Could you check a few things on this model? Use its own coordinates, in mm. A direction names the side the tool comes from. Round coordinates to 2 decimals unless told otherwise and drop trailing zeros. Loops run counter-clockwise (first coordinate to the right, second up) from the corner with the lowest first, then second, coordinate; pieces in that order, holes last. Notation, with made-up numbers: (4.5, 85.5) -> (51.5, 85.5) arc R21 ccw to (51.5, 113.5) -> close; hole circle Ø10 at (34, -19). An arc over 180 degrees is marked (long way). Write each question's results on one line, items separated by ' | '.
from build123d import *

# Parameters (mm, degrees)
F1_DEPTH = 7.62
F2_DEPTH = 25.4
F4_DEPTH = 25.4
F6_DEPTH = 25.4


with BuildPart() as f1:
    # F0 (on Front) → F1 (new body)
    with BuildSketch(Plane.XZ):
        Polygon((0, -4.6985740773), (0, 0), (-4.4972063042, 0), (-18.1230716407, 0), align=None)
        Polygon((4.698574543, 0), (0, 0), (0, -4.6985740773), (4.698574543, -4.6985740773), (18.9285408705, 0), (10.8738420531, 0), align=None)
        Polygon((-4.4972063042, 0), (0, 0), (4.698574543, 0), (4.698574543, 44.1665910184), (0, 56.5171316266), (-4.4972063042, 43.0926345289), (-4.4972063042, 26.4462586492), align=None)
        with BuildLine():
            Line((4.698574543, -4.6985740773), (0, -4.6985740773))
            Line((0, -4.6985740773), (-4.4972063042, -4.6985740773))
            Line((-4.4972063042, -4.6985740773), (-4.4972063042, -7.9204533249))
            add(Edge.make_bspline(
                [(-4.4972063042, -7.9204533249), (-3.0188959312, -8.9298356018), (-0.076765682, -10.9387061232), (3.1120295895, -9.4610912419), (4.698574543, -8.7259225547)],
                knots=[0, 0, 0, 0, 0.5024625859, 1, 1, 1, 1], degree=3))
            Line((4.698574543, -8.7259225547), (4.698574543, -4.6985740773))
        make_face()
        Polygon((-4.4972063042, -4.6985740773), (0, -4.6985740773), (-18.1230716407, 0), (-8.9944126084, -4.6985740773), align=None)
        Polygon((18.9285408705, 0), (4.698574543, -4.6985740773), (10.8738420531, -4.6985740773), align=None)
        with BuildLine():
            add(Edge.make_bspline(
                [(-4.4972063042, -7.9204533249), (-3.0188959312, -8.9298356018), (-0.076765682, -10.9387061232), (3.1120295895, -9.4610912419), (4.698574543, -8.7259225547)],
                knots=[0, 0, 0, 0, 0.5024625859, 1, 1, 1, 1], degree=3))
            Line((-4.4972063042, -7.9204533249), (-4.4972063042, -12.2162923217))
            add(Edge.make_bspline(
                [(-4.4972063042, -12.2162923217), (-3.0081701645, -13.4176450734), (-0.0043271069, -15.841142413), (3.1220001254, -13.4314667708), (4.698574543, -12.2162923217)],
                knots=[0, 0, 0, 0, 0.4957103654, 1, 1, 1, 1], degree=3))
            Line((4.698574543, -12.2162923217), (4.698574543, -8.7259225547))
        make_face()
        with BuildLine():
            add(Edge.make_bspline(
                [(-4.4972063042, -12.2162923217), (-3.0081701645, -13.4176450734), (-0.0043271069, -15.841142413), (3.1220001254, -13.4314667708), (4.698574543, -12.2162923217)],
                knots=[0, 0, 0, 0, 0.4957103654, 1, 1, 1, 1], degree=3))
            Line((-4.4972063042, -12.2162923217), (-4.4972063042, -17.720336793))
            add(Edge.make_bspline(
                [(-4.4972063042, -17.720336793), (-3.009588296, -19.5245403943), (-0.0141265995, -23.1574775803), (3.1206187826, -19.5408569928), (4.698574543, -17.720336793)],
                knots=[0, 0, 0, 0, 0.4966239461, 1, 1, 1, 1], degree=3))
            Line((4.698574543, -17.720336793), (4.698574543, -12.2162923217))
        make_face()
        with BuildLine():
            add(Edge.make_bspline(
                [(-4.4972063042, -17.720336793), (-3.009588296, -19.5245403943), (-0.0141265995, -23.1574775803), (3.1206187826, -19.5408569928), (4.698574543, -17.720336793)],
                knots=[0, 0, 0, 0, 0.4966239461, 1, 1, 1, 1], degree=3))
            Line((-4.4972063042, -17.720336793), (-4.4972063042, -24.8353201896))
            add(Edge.make_bspline(
                [(-4.4972063042, -24.8353201896), (-3.0004006611, -25.540556717), (0.0506661056, -26.9781005566), (3.1299428272, -25.2027364557), (4.698574543, -24.2983382195)],
                knots=[0, 0, 0, 0, 0.490584362, 1, 1, 1, 1], degree=3))
            Line((4.698574543, -24.2983382195), (4.698574543, -17.720336793))
        make_face()
        with BuildLine():
            add(Edge.make_bspline(
                [(-4.4972063042, -24.8353201896), (-3.0004006611, -25.540556717), (0.0506661056, -26.9781005566), (3.1299428272, -25.2027364557), (4.698574543, -24.2983382195)],
                knots=[0, 0, 0, 0, 0.490584362, 1, 1, 1, 1], degree=3))
            Line((-4.4972063042, -24.8353201896), (-4.4972063042, -30.7420995086))
            Line((-4.4972063042, -30.7420995086), (0, -30.7420995086))
            Line((0, -30.7420995086), (4.698574543, -30.7420995086))
            Line((4.698574543, -30.7420995086), (4.698574543, -24.2983382195))
        make_face()
    extrude(amount=F1_DEPTH)

    # F2 (add): a face of the model
    f2_faces = [f1.faces().sort_by_distance(p)[0] for p in [
        (0.1945490667, -7.62, 8.4784905135),
    ]]
    extrude(f2_faces, amount=F2_DEPTH)

    # F3 (on face) → F4 (cut)
    with BuildSketch(Plane.XZ.offset(33.02)):
        Polygon((-8.9944126084, -4.6985740773), (-4.4972063042, -4.6985740773), (-4.4972063042, -30.7420995086), (4.698574543, -30.7420995086), (4.698574543, -4.6985740773), (10.8738420531, -4.6985740773), (18.9285408705, 0), (4.698574543, 0), (4.698574543, 44.1665910184), (0, 56.5171316266), (-4.4972063042, 43.0926345289), (-4.4972063042, 0), (-18.1230716407, 0), align=None)
    extrude(amount=-F4_DEPTH, mode=Mode.SUBTRACT)

    # F5 (on Front) → F6 (join)
    with BuildSketch(Plane.XZ):
        with BuildLine():
            ThreePointArc((-17.5860915333, 4.6985740773), (-21.4011571542, 3.3053396825), (-23.7613599747, 0))
            ThreePointArc((-23.7613599747, 0), (-17.0294068149, -9.0208482643), (-10.8738420531, 0.4027348768))
            ThreePointArc((-10.8738420531, 0.4027348768), (-13.5428980412, 3.6241995188), (-17.5860915333, 4.6985740773))
        make_face()
    extrude(amount=F6_DEPTH)


solid = f1.part
1) For faces 4 (the flat face through (-4.497, -4, -18)), 5 (the flat face through (-8, -4, 0)), 6 (the flat face through (8, -4, -4.699)), 7 (the flat face through (4.699, -4, 22)), which set-ups out of +Z, -Z, +X, -X, +Y, -Y let a thin tool reach every point of the face, with its end or its side?
Model answer:
face 4: -Z, +Y, -Y | face 5: +Z, +Y, -Y | face 6: -Z, +X, +Y, -Y | face 7: +Z, +X, +Y, -Y
2) I want a section at D-D, the plane y = -15.5. Write out the boundary of the cut face in (x, z).
Model answer:
outline: circle Ø13.73 at (-17.24, -2.16)
3) I want a section at A-A, the plane y = -5.5. Write out the boundary of the cut face in (x, z), plus the area to 3 significant figures.
Model answer:
outline: (-10.73, 0) arc R6.87 ccw (long way) to (-10.6, -3.87) -> (-8.99, -4.7) -> (-4.5, -4.7) -> (-4.5, -30.74) -> (4.7, -30.74) -> (4.7, -4.7) -> (10.87, -4.7) -> (18.93, 0) -> (4.7, 0) -> (4.7, 44.17) -> (0, 56.52) -> (-4.5, 43.09) -> (-4.5, 0) -> close | area: 967 mm2
4) I want a section at C-C, the plane z = 33.5. Write out the boundary of the cut face in (x, y).
Model answer:
outline: (-4.5, -7.62) -> (4.7, -7.62) -> (4.7, 0) -> (-4.5, 0) -> close
5) If we mould it in two halves opening along X, with no side actions, what happens to faces 1 (the flat face through (-7, -4, -4.699)), 2 (the flat face through (4.699, -4, -18)), 3 (the flat face through (0, -4, -30.742))? For each: released by +X, released by -X, zero draft, split by the parting line, or undercut.
Model answer:
face 1: undercut | face 2: released by +X | face 3: zero draft
6) I need wall thicknesses on line 1 (X direction, y = -2.5, z = 13.5); line 2 (Y direction, x = 0, z = -13); line 3 (X direction, y = -16.25, z = 3). Which ranges of each line are inside material? Lowest first, please.
Model answer:
line 1: x = -4.5 to 4.7 | line 2: y = -7.62 to 0 | line 3: x = -21.77 to -12.71
7) I want a section at B-B, the plane x = -7. Write out the boundary of the cut face in (y, z), plus the area to 3 significant figures.
Model answer:
outline: (-7.62, -4.7) -> (0, -4.7) -> (0, 0) -> (-7.62, 0) -> close | area: 35.8 mm2
8) I'm going to push flat-ended pins straight in: pin 1 (6 mm diameter, centred on x = 13.5, y = -5, fed in from +Z); pin 2 (6 mm diameter, centred on y = -5, z = 22.5, fed in from -X); pin 3 (1.9 mm diameter, centred on x = 8.5, y = -3, fed in from -Z); pin 4 (4 mm diameter, centred on x = 13, y = -11, fed in from +Z). Where does each tip first touch, or does it pass through?
Model answer:
pin 1: stops at z = 0 | pin 2: stops at x = -4.5 | pin 3: stops at z = -4.7 | pin 4: passes through
